from build123d import *

# Parameters (mm, degrees)
SKETCH_1_R               = 61
EXTRUDE_1_DEPTH          = 2
PATTERN_CIRCULAR_1_COUNT = 4
HOLE_WIZARD_M3_1_D       = 2.5
PATTERN_CIRCULAR_2_COUNT = 4
HOLE_WIZARD_M3_2_D       = 2.5
HOLE_WIZARD_M3_3_D       = 2.5


with BuildPart() as part:
    # 草图1 → 凸台-拉伸1 (new body)
    with BuildSketch(Plane.XY):
        Circle(SKETCH_1_R)
    extrude(amount=EXTRUDE_1_DEPTH)

    # 草图3 → 打孔尺寸(%根据十字)槽半沉头木螺钉的类型1 (revolve, cut)
    with BuildSketch(Plane(origin=(0, 57, 2), x_dir=(0, -1, 0), z_dir=(1, 0, 0))):
        Polygon((0, 0), (0, 2), (1.7, 2), (1.7, 1.6), (3.3, 0), align=None)
    hole_wizard_1 = revolve(axis=Axis((0, 57, 8.35), (0, 0, -1)), mode=Mode.SUBTRACT)

    # 阵列(圆周)1: 打孔尺寸(%根据十字)槽半沉头木螺钉的类型1 ×4 about axis
    pattern_circular_1_axis = Axis((0, 0, 0), (0, 0, 1))
    for i in range(1, PATTERN_CIRCULAR_1_COUNT):
        add(hole_wizard_1.rotate(pattern_circular_1_axis, i * 360 / PATTERN_CIRCULAR_1_COUNT), mode=Mode.SUBTRACT)

    # M3 螺纹孔1 (through all)
    with Locations(Plane(origin=(0, 0, 0), x_dir=(-1, 0, 0), z_dir=(0, 0, -1))):
        with Locations((-20, 0)):
            hole_wizard_m3_1 = Hole(HOLE_WIZARD_M3_1_D / 2)

    # 阵列(圆周)2: M3 螺纹孔1 ×4 about axis
    pattern_circular_2_axis = Axis((0, 0, 0), (0, 0, 1))
    for i in range(1, PATTERN_CIRCULAR_2_COUNT):
        add(hole_wizard_m3_1.rotate(pattern_circular_2_axis, i * 360 / PATTERN_CIRCULAR_2_COUNT), mode=Mode.SUBTRACT)

    # M3 螺纹孔2 (through all)
    with Locations(Plane(origin=(0, 0, 0), x_dir=(-1, 0, 0), z_dir=(0, 0, -1))):
        with Locations((0, 0)):
            Hole(HOLE_WIZARD_M3_2_D / 2)

    # M3 螺纹孔3 (through all)
    with Locations(Plane(origin=(0, 0, 0), x_dir=(-1, 0, 0), z_dir=(0, 0, -1))):
        with Locations((34.387640449, -28.244294722), (44.5, 0)):
            Hole(HOLE_WIZARD_M3_3_D / 2)


solid = part.part
Work out the finished part from the listing and answer in its coordinate system (mm). Round coordinates to 2 decimals unless told otherwise and drop trailing zeros. Write each loop counter-clockwise with the first axis right and the second up, starting at its lowest first coordinate (ties: lowest second). Pieces come first, ordered by that corner, then holes. Notation, with made-up numbers: (62.5, 37) - (120.5, 37) arc R22 cw to (120.5, 58) - close; hole circle Ø5 at (-20.75, 16.5). An arc over 180 degrees is marked (long way). Answer in a Markdown table with one row per item. Add a question column.
1. A cutting plane is placed at B-B, the plane x = -57. Determine the outline of the cut face in (y, z), and give its area (3 significant figures).
2. A cutting plane is placed at D-D, the plane x = -16. Determine the outline of the cut face in (y, z), and give its area (3 significant figures).
3. Given pin 1 (2 mm diameter, centred on x = -57, y = 0, fed in from +Z); pin 2 (4.5 mm diameter, centred on x = 0, y = 57, fed in from +Z); pin 3 (5.5 mm diameter, centred on x = 57, y = 0, fed in from +Z), each flat-ended and moving along its own axis, determine where each tip first touches the part or whether it passes through.
4. A cutting plane is placed at A-A, the plane z = 1.35. Count the separate pieces of the cut face and the enclosed holes in it, and give its area (3 significant figures).
5. The mould has two halves that part along X. Classify faces 1 (the cylindrical face through (-58.7, -0.07, 0.2)), 2 (the cylindrical face through (-48.408, -37.118, 0.986)), 3 (the flat face through (-1, -13, 2)): +X half, -X half, draft (parallel to the pull), parting line (faces both ways), or undercut.
6. Find the intervals of material crossed by line 1 along Y through (x, z) = (1.5, 0.1); line 2 along Y through (x, z) = (-20, 1.25); line 3 along Y through (x, z) = (-39, 1.9), in increasing order. Write a range as from..to.
Worked out:
| question | item | result |
|---|---|---|
| 1 | outline | (-21.73, 0) - (-1.7, 0) - (-1.7, 0.4) - (-3.3, 2) - (-21.73, 2) - close; (1.7, 0) - (21.73, 0) - (21.73, 2) - (3.3, 2) - (1.7, 0.4) - close |
| 1 | area | 77.5 mm^2 |
| 2 | outline | (-58.86, 0) - (58.86, 0) - (58.86, 2) - (-58.86, 2) - close |
| 2 | area | 235 mm^2 |
| 3 | pin 1 | through |
| 3 | pin 2 | z = 0.95 |
| 3 | pin 3 | z = 1.45 |
| 4 | separate pieces | 1 |
| 4 | enclosed holes | 11 |
| 4 | area | 11,600 mm^2 |
| 5 | face 1 | undercut |
| 5 | face 2 | parting line |
| 5 | face 3 | draft |
| 6 | line 1 | -60.98..-57.8, -56.2..56.2, 57.8..60.98 |
| 6 | line 2 | -57.63..-1.25, 1.25..57.63 |
| 6 | line 3 | -46.9..46.9 |
